The listing builds one solid part. Answer for the finished solid, in the listing's coordinates (mm). Face numbers are marked on the shaded views. Round coordinates to 2 decimals unless told otherwise and drop trailing zeros. Order: outer loops, then holes, each group sorted by start corner. A loop starts at its lowest first (then second) coordinate and runs counter-clockwise, first axis right, second up. Notation, with made-up numbers: (49, 71.25) - (61, 71.25) arc R35 cw to (61, 108.25) - close; hole circle Ø11 at (-19, 48). An arc over 180 degrees is marked (long way). Write item = value, one per line.
from build123d import *

# Parameters (mm, degrees)
SKETCH1_W                 = 190
SKETCH1_H                 = 55
SKETCH1_R                 = 2
BOSS_EXTRUDE1_DEPTH       = 2
SKETCH2_W                 = 10
SKETCH2_H                 = 10
BOSS_EXTRUDE2_DEPTH       = 7.1
LPATTERN1_COUNT           = 2
LPATTERN1_PITCH           = 22.5
SKETCH3_W                 = 8
SKETCH3_H                 = 3
CUT_EXTRUDE1_DEPTH        = 7.1
LPATTERN2_COUNT           = 3
LPATTERN2_PITCH           = 22.5
SKETCH4_W                 = 2
SKETCH4_H                 = 6
CUT_EXTRUDE2_DEPTH        = 7.1
LPATTERN3_COUNT           = 3
LPATTERN3_PITCH           = 15
LPATTERN4_COUNT           = 4
LPATTERN4_PITCH           = 20
LPATTERN4_COPY_1_SKETCH_W = 2
LPATTERN4_COPY_1_SKETCH_H = 6
LPATTERN4_COPY_1_DEPTH    = 7.1
LPATTERN4_COPY_2_SKETCH_W = 2
LPATTERN4_COPY_2_SKETCH_H = 6
LPATTERN4_COPY_2_DEPTH    = 7.1
LPATTERN4_COPY_3_SKETCH_W = 2
LPATTERN4_COPY_3_SKETCH_H = 6
LPATTERN4_COPY_3_DEPTH    = 7.1
LPATTERN4_COPY_4_SKETCH_W = 2
LPATTERN4_COPY_4_SKETCH_H = 6
LPATTERN4_COPY_4_DEPTH    = 7.1
LPATTERN4_COPY_5_SKETCH_W = 2
LPATTERN4_COPY_5_SKETCH_H = 6
LPATTERN4_COPY_5_DEPTH    = 7.1
LPATTERN4_COPY_6_SKETCH_W = 2
LPATTERN4_COPY_6_SKETCH_H = 6
LPATTERN4_COPY_6_DEPTH    = 7.1
SKETCH5_W                 = 10
SKETCH5_H                 = 10
BOSS_EXTRUDE3_DEPTH       = 7.1


with BuildPart() as part:
    # Sketch1 → Boss-Extrude1 (new body)
    with BuildSketch(Plane(origin=(0, 0, 0), x_dir=(1, 0, 0), z_dir=(0, 1, 0))):
        with Locations((75, 22.5)):
            Rectangle(SKETCH1_W, SKETCH1_H)
        Circle(SKETCH1_R, mode=Mode.SUBTRACT)
        with Locations((25, 0)):
            Circle(SKETCH1_R, mode=Mode.SUBTRACT)
        with Locations((50, 0)):
            Circle(SKETCH1_R, mode=Mode.SUBTRACT)
        with Locations((75, 0)):
            Circle(SKETCH1_R, mode=Mode.SUBTRACT)
        with Locations((100, 0)):
            Circle(SKETCH1_R, mode=Mode.SUBTRACT)
        with Locations((125, 0)):
            Circle(SKETCH1_R, mode=Mode.SUBTRACT)
        with Locations((150, 0)):
            Circle(SKETCH1_R, mode=Mode.SUBTRACT)
    extrude(amount=BOSS_EXTRUDE1_DEPTH)

    # Sketch2 → Boss-Extrude2 (add)
    with BuildSketch(Plane.XZ):
        with Locations((125, -22.5)):
            Rectangle(SKETCH2_W, SKETCH2_H)
    boss_extrude2 = extrude(amount=BOSS_EXTRUDE2_DEPTH)

    # LPattern1: Boss-Extrude2 ×2
    with Locations(*[(0, 0, -i * LPATTERN1_PITCH) for i in range(1, LPATTERN1_COUNT)]):
        add(boss_extrude2)

    # Sketch3 → Cut-Extrude1 (cut)
    with BuildSketch(Plane(origin=(0, 2, 0), x_dir=(1, 0, 0), z_dir=(0, 1, 0))):
        with Locations((160, 30.5)):
            Rectangle(SKETCH3_W, SKETCH3_H)
        with Locations((160, 14.5)):
            Rectangle(SKETCH3_W, SKETCH3_H)
    cut_extrude1 = extrude(amount=-CUT_EXTRUDE1_DEPTH, mode=Mode.SUBTRACT)

    # LPattern2: Cut-Extrude1 ×3
    with Locations(*[(-i * LPATTERN2_PITCH, 0, 0) for i in range(1, LPATTERN2_COUNT)]):
        add(cut_extrude1, mode=Mode.SUBTRACT)

    # Sketch4 → Cut-Extrude2 (cut)
    with BuildSketch(Plane(origin=(0, 2, 0), x_dir=(1, 0, 0), z_dir=(0, 1, 0))):
        with Locations((-5, 10)):
            Rectangle(SKETCH4_W, SKETCH4_H)
        with Locations((5, 10)):
            Rectangle(SKETCH4_W, SKETCH4_H)
    cut_extrude2 = extrude(amount=-CUT_EXTRUDE2_DEPTH, mode=Mode.SUBTRACT)

    # LPattern3: Cut-Extrude2 ×3
    with Locations(*[(0, 0, -i * LPATTERN3_PITCH) for i in range(1, LPATTERN3_COUNT)]):
        add(cut_extrude2, mode=Mode.SUBTRACT)

    # LPattern4: Cut-Extrude2 ×4
    with Locations(*[(i * LPATTERN4_PITCH, 0, 0) for i in range(1, LPATTERN4_COUNT)]):
        add(cut_extrude2, mode=Mode.SUBTRACT)

    # LPattern4 copy 1 sketch → LPattern4 copy 1 (cut)
    with BuildSketch(Plane(origin=(20, 2, -15), x_dir=(1, 0, 0), z_dir=(0, 1, 0))):
        with Locations((-5, 10)):
            Rectangle(LPATTERN4_COPY_1_SKETCH_W, LPATTERN4_COPY_1_SKETCH_H)
        with Locations((5, 10)):
            Rectangle(LPATTERN4_COPY_1_SKETCH_W, LPATTERN4_COPY_1_SKETCH_H)
    extrude(amount=-LPATTERN4_COPY_1_DEPTH, mode=Mode.SUBTRACT)

    # LPattern4 copy 2 sketch → LPattern4 copy 2 (cut)
    with BuildSketch(Plane(origin=(40, 2, -15), x_dir=(1, 0, 0), z_dir=(0, 1, 0))):
        with Locations((-5, 10)):
            Rectangle(LPATTERN4_COPY_2_SKETCH_W, LPATTERN4_COPY_2_SKETCH_H)
        with Locations((5, 10)):
            Rectangle(LPATTERN4_COPY_2_SKETCH_W, LPATTERN4_COPY_2_SKETCH_H)
    extrude(amount=-LPATTERN4_COPY_2_DEPTH, mode=Mode.SUBTRACT)

    # LPattern4 copy 3 sketch → LPattern4 copy 3 (cut)
    with BuildSketch(Plane(origin=(60, 2, -15), x_dir=(1, 0, 0), z_dir=(0, 1, 0))):
        with Locations((-5, 10)):
            Rectangle(LPATTERN4_COPY_3_SKETCH_W, LPATTERN4_COPY_3_SKETCH_H)
        with Locations((5, 10)):
            Rectangle(LPATTERN4_COPY_3_SKETCH_W, LPATTERN4_COPY_3_SKETCH_H)
    extrude(amount=-LPATTERN4_COPY_3_DEPTH, mode=Mode.SUBTRACT)

    # LPattern4 copy 4 sketch → LPattern4 copy 4 (cut)
    with BuildSketch(Plane(origin=(20, 2, -30), x_dir=(1, 0, 0), z_dir=(0, 1, 0))):
        with Locations((-5, 10)):
            Rectangle(LPATTERN4_COPY_4_SKETCH_W, LPATTERN4_COPY_4_SKETCH_H)
        with Locations((5, 10)):
            Rectangle(LPATTERN4_COPY_4_SKETCH_W, LPATTERN4_COPY_4_SKETCH_H)
    extrude(amount=-LPATTERN4_COPY_4_DEPTH, mode=Mode.SUBTRACT)

    # LPattern4 copy 5 sketch → LPattern4 copy 5 (cut)
    with BuildSketch(Plane(origin=(40, 2, -30), x_dir=(1, 0, 0), z_dir=(0, 1, 0))):
        with Locations((-5, 10)):
            Rectangle(LPATTERN4_COPY_5_SKETCH_W, LPATTERN4_COPY_5_SKETCH_H)
        with Locations((5, 10)):
            Rectangle(LPATTERN4_COPY_5_SKETCH_W, LPATTERN4_COPY_5_SKETCH_H)
    extrude(amount=-LPATTERN4_COPY_5_DEPTH, mode=Mode.SUBTRACT)

    # LPattern4 copy 6 sketch → LPattern4 copy 6 (cut)
    with BuildSketch(Plane(origin=(60, 2, -30), x_dir=(1, 0, 0), z_dir=(0, 1, 0))):
        with Locations((-5, 10)):
            Rectangle(LPATTERN4_COPY_6_SKETCH_W, LPATTERN4_COPY_6_SKETCH_H)
        with Locations((5, 10)):
            Rectangle(LPATTERN4_COPY_6_SKETCH_W, LPATTERN4_COPY_6_SKETCH_H)
    extrude(amount=-LPATTERN4_COPY_6_DEPTH, mode=Mode.SUBTRACT)

    # Sketch5 → Boss-Extrude3 (add)
    with BuildSketch(Plane.XZ):
        with Locations((-15, -45)):
            Rectangle(SKETCH5_W, SKETCH5_H)
        with Locations((-15, -20)):
            Rectangle(SKETCH5_W, SKETCH5_H)
    extrude(amount=BOSS_EXTRUDE3_DEPTH)


solid = part.part
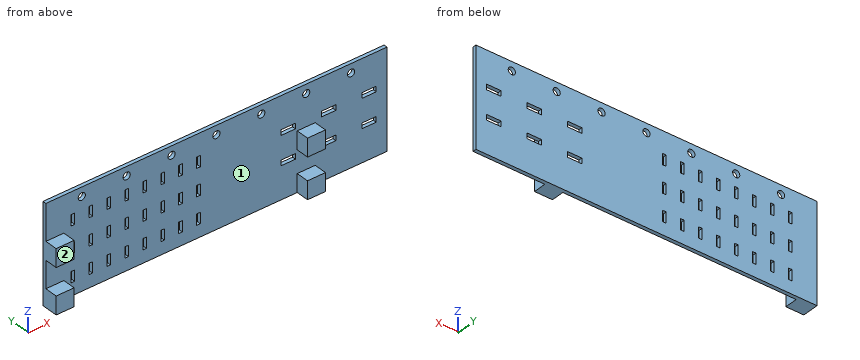
Q1. Section A-A on x = 100 is taken. Determine the outline of the cut face in (y, z), then the cut area to 3 significant figures.
Model answer:
outline = (0, -50) - (2, -50) - (2, -2) - (0, -2) - close; (0, 2) - (2, 2) - (2, 5) - (0, 5) - close
area = 102 mm^2
Q2. Determine the mould class of the marked faces 1 and 2 for opening direction X: released by +X, released by -X, zero draft, split by the parting line, or undercut.
Model answer:
face_1 = undercut
face_2 = zero draft
Q3. Flat-ended cylindrical pins translate along their axes: P1, Ø3.5, axis at y = -4.5, z = -24, coming from the +X side; P2, Ø6.5, axis at x = 100, z = 0, coming from the +Y side; P3, Ø12, axis at x = 106, z = -23, coming from the -Y side. Find the tip coordinate at first contact, or state that the pin passes through.
Model answer:
P1 = 130
P2 = 2
P3 = 0
Q4. Section B-B on y = -2.5 is taken. Determine the outline of the cut face in (x, z).
Model answer:
outline = (-20, -50) - (-10, -50) - (-10, -40) - (-20, -40) - close; (-20, -25) - (-10, -25) - (-10, -15) - (-20, -15) - close; (120, -50) - (130, -50) - (130, -40) - (120, -40) - close; (120, -27.5) - (130, -27.5) - (130, -17.5) - (120, -17.5) - close
Q5. Find the intervals of material crossed by line 1 (Z direction, x = 160.5, y = 0.25); line 2 (Z direction, x = 0, y = 0.7); line 3 (Z direction, x = 25, y = 0.9), in increasing order. Write a range as from..to.
Model answer:
line_1 = -50..-32, -29..-16, -13..5
line_2 = -50..-2, 2..5
line_3 = -50..-43, -37..-28, -22..-13, -7..-2, 2..5
